Read the model definition and answer for the solid it produces. Units are mm, in the model's axes. Face numbers are marked on the shaded views. A direction names the side the tool comes from. Coordinates: 2 decimals unless noted, no trailing zeros. Loops run counter-clockwise (first coordinate to the right, second up) from the corner with the lowest first, then second, coordinate; pieces in that order, holes last.
from build123d import *

# Parameters (mm, degrees)
SKETCH1_W           = 44
SKETCH1_H           = 19.5
BOSS_EXTRUDE1_DEPTH = 6.5
CUT_EXTRUDE1_REACH  = 50.564
SKETCH2_W           = 10
SKETCH2_H           = 6.5
FILLET1_R           = 8
CUT_EXTRUDE2_REACH  = 50.564
SKETCH3_R           = 2.5


with BuildPart() as part:
    # Sketch1 → Boss-Extrude1 (new body)
    with BuildSketch(Plane.XY):
        with Locations((22, 9.75)):
            Rectangle(SKETCH1_W, SKETCH1_H)
    extrude(amount=BOSS_EXTRUDE1_DEPTH)

    # Sketch2 → Cut-Extrude1 (cut, up to next)
    with BuildSketch(Plane.XY.offset(6.5), mode=Mode.PRIVATE) as cut_extrude1_sk1:
        with Locations((29, 16.25)):
            Rectangle(SKETCH2_W, SKETCH2_H)
    cut_extrude1_tool1 = extrude(cut_extrude1_sk1.sketch, amount=-CUT_EXTRUDE1_REACH, mode=Mode.PRIVATE) & part.part
    # Sketch2 → Cut-Extrude1 (cut, up to next)
    with BuildSketch(Plane.XY.offset(6.5), mode=Mode.PRIVATE) as cut_extrude1_sk2:
        with Locations((29, 3.25)):
            Rectangle(SKETCH2_W, SKETCH2_H)
    cut_extrude1_tool2 = extrude(cut_extrude1_sk2.sketch, amount=-CUT_EXTRUDE1_REACH, mode=Mode.PRIVATE) & part.part
    add(cut_extrude1_tool1.solids().sort_by_distance((29, 16.25, 6.5))[0], mode=Mode.SUBTRACT)
    add(cut_extrude1_tool2.solids().sort_by_distance((29, 3.25, 6.5))[0], mode=Mode.SUBTRACT)

    # Fillet1
    fillet1_edges = [part.edges().sort_by_distance(p)[0] for p in [
        (0, 19.5, 3.25),
        (0, 0, 3.25),
    ]]
    fillet(fillet1_edges, radius=FILLET1_R)

    # Sketch3 → Cut-Extrude2 (cut, up to next)
    with BuildSketch(Plane.XY.offset(6.5), mode=Mode.PRIVATE) as cut_extrude2_sk1:
        with Locations((10, 10.072944896)):
            Circle(SKETCH3_R)
    cut_extrude2_tool1 = extrude(cut_extrude2_sk1.sketch, amount=-CUT_EXTRUDE2_REACH, mode=Mode.PRIVATE) & part.part
    add(cut_extrude2_tool1.solids().sort_by_distance((10, 10.072945, 6.5))[0], mode=Mode.SUBTRACT)


solid = part.part
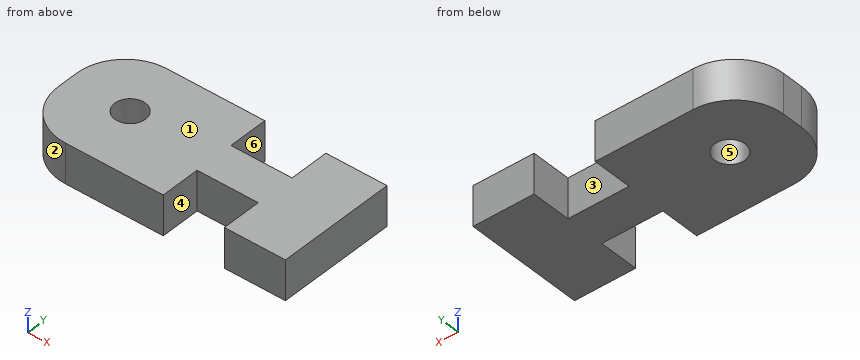
Q1. A cutting plane is placed at B-B (y = 1.5). Give the vertices of the cut face in (x, z), then the cut area to 3 significant figures.
Findings below:
outline: (3.34, 0) - (24, 0) - (24, 6.5) - (3.34, 6.5) - close; (34, 0) - (44, 0) - (44, 6.5) - (34, 6.5) - close
area: 199 mm2
Q2. Flat-ended cylindrical pins translate along their axes: pin 1 Ø2 at (y, z) = (17.5, 4.5) entering from -X (3 decimals); pin 2 Ø2 at (y, z) = (4.5, 1.5) entering from -X; pin 3 Ø1.5 at (x, z) = (31, 1.5) entering from -Y. Find the tip coordinate at first contact, or state that the pin passes through.
Findings below:
pin 1: stops at x = 1.755
pin 2: stops at x = 0.4
pin 3: stops at y = 6.5
Q3. Which of the six approach directions +Z, -Z, +X, -X, +Y, -Y give full straight-line access (tool end or side, diameter ignored) to the marked faces 4, 5 and 6?
Findings below:
face 4: +Z, -Z, -Y
face 5: +Z, -Z
face 6: +Z, -Z, +Y
Q4. Determine the mould class of the marked faces 1, 2 and 3 for opening direction X: +X half, -X half, draft (parallel to the pull), parting line (faces both ways), or undercut.
Findings below:
face 1: draft
face 2: -X half
face 3: undercut
Q5. Straight lines are drawn through the part: probe 1 along Y at (x, z) = (10, 2); probe 2 along X at (y, z) = (10, 4.5); probe 3 along X at (y, z) = (2, 4.5). For each, find the intervals that lie inside material, in ascending order.
Findings below:
probe 1: y = 0 to 7.57, 12.57 to 19.5
probe 2: x = 0 to 7.5, 12.5 to 44
probe 3: x = 2.71 to 24, 34 to 44
Q6. A cutting plane is placed at A-A (x = 10). Give the vertices of the cut face in (y, z).
Findings below:
outline: (0, 0) - (7.57, 0) - (7.57, 6.5) - (0, 6.5) - close; (12.57, 0) - (19.5, 0) - (19.5, 6.5) - (12.57, 6.5) - close
Q7. A cutting plane is placed at D-D (x = 28). Give the vertices of the cut face in (y, z).
Findings below:
outline: (6.5, 0) - (13, 0) - (13, 6.5) - (6.5, 6.5) - close
Q8. A cutting plane is placed at C-C (z = 3.5). Give the vertices of the cut face in (x, y), then the cut area to 3 significant figures.
Findings below:
outline: (0, 8) arc R8 ccw to (8, 0) - (24, 0) - (24, 6.5) - (34, 6.5) - (34, 0) - (44, 0) - (44, 19.5) - (34, 19.5) - (34, 13) - (24, 13) - (24, 19.5) - (8, 19.5) arc R8 ccw to (0, 11.5) - close; hole circle Ø5 at (10, 10.07)
area: 681 mm2
